Work out the finished part from the listing and answer in its coordinate system (mm). A direction names the side the tool comes from. Give positions to 0.01 mm unless a question says otherwise; leave off trailing zeros. Loops run counter-clockwise (first coordinate to the right, second up) from the corner with the lowest first, then second, coordinate; pieces in that order, holes last.
```python
from build123d import *

# Parameters (mm, degrees)
F0_W      = 60
F0_H      = 10
F1_DEPTH  = 60
F2_SIZE   = 9.99999
F9_DEPTH  = 40
F11_DEPTH = 20
F13_R     = 15
F14_DEPTH = 26
F15_R     = 2


# Not quite as in the source:
# - a fillet or chamfer is up to 0.001 mm smaller than in the source, because OpenCascade refuses the exact size


with BuildPart() as f1:
    # F0 (on Front) → F1 (new body)
    with BuildSketch(Plane.XZ):
        with Locations((30, 5)):
            Rectangle(F0_W, F0_H)
    extrude(amount=-F1_DEPTH)

    # F2 (size 10 in the source; OpenCascade refuses exactly that, so slightly less here)
    f2_edges = [f1.edges().sort_by_distance(p)[0] for p in [
        (60, 30, 0),
    ]]
    chamfer(f2_edges, length=F2_SIZE)

    # F5 (on face) → F6 section 0
    with BuildSketch(Plane.XY.offset(10), mode=Mode.PRIVATE) as f6_s0:
        Polygon((60, 0), (60, 60), (0, 0), align=None)
    loft([f6_s0.sketch, Vertex(60, 60, 70)])

    # F8 (on face) → F9 (join)
    with BuildSketch(Plane.XY.offset(10)):
        Polygon((40, 60), (0, 60), (0, 20), align=None)
    extrude(amount=F9_DEPTH)

    # F10 (on face) → F11 (join)
    with BuildSketch(Plane(origin=(0, 0, 0), x_dir=(1, 0, 0), z_dir=(0, 0, -1))):
        Polygon((0, -20), (0, -60), (40, -60), align=None)
    extrude(amount=F11_DEPTH)

    # F9_face (on face) → F12 section 0
    with BuildSketch(Plane(origin=(13.3333333333, 46.6666666667, 50), x_dir=(1, 0, 0), z_dir=(0, 0, 1)), mode=Mode.PRIVATE) as f12_s0:
        Polygon((26.6666666667, 13.3333333333), (-13.3333333333, 13.3333333333), (-13.3333333333, -26.6666666667), align=None)
    loft([f12_s0.sketch, Vertex(0, 60, -20)], mode=Mode.SUBTRACT)

    # F13 (on face) → F14 (cut)
    with BuildSketch(Plane(origin=(0, 0, -20), x_dir=(1, 0, 0), z_dir=(0, 0, -1))):
        with Locations((30, -40)):
            Circle(F13_R)
    extrude(amount=-F14_DEPTH, mode=Mode.SUBTRACT)

    # F15
    f15_edges = [f1.edges().sort_by_distance(p)[0] for p in [
        (15, 40, 6),
    ]]
    fillet(f15_edges, radius=F15_R)


solid = f1.part
```
Q1. Section C-C on x = 30 is taken. Give the vertices of the cut face in (y, z).
Q2. Consider line 1 along Y through (x, z) = (30, -13); line 2 along X through (y, z) = (22, 24.5); line 3 along Z through (x, y) = (12, 52). Determine where each line is inside the solid, lowest interval first.
Q3. Section A-A on y = 4 is taken. Give the vertices of the cut face in (x, z), plus the area to 3 significant figures.
Q4. Section D-D on z = 36.5 is taken. Give the vertices of the cut face in (x, y), plus the area to 3 significant figures.
Q5. Given pin 1 (4 mm diameter, centred on x = 30.5, y = 37.5, fed in from -Z); pin 2 (4 mm diameter, centred on x = 24, z = 14, fed in from -Y); pin 3 (12 mm diameter, centred on x = 19, z = 55, fed in from +Y), each flat-ended and moving along its own axis, determine where each tip first touches the part or whether it passes through.
Q6. Section B-B on z = 8 is taken. Give the vertices of the cut face in (x, y), plus the area to 3 significant figures.
Q7. Which of the six approach directions +Z, -Z, +X, -X, +Y, -Y give full straight-line access (tool end or side, diameter ignored) to faces 5 (the face through (8, 28, -10)), 6 (the face through (60, 43, 27)), 7 (the face through (43, 17, 27)), 8 (the face through (44, 44, 27)), 9 (the face through (18, 49, -6))?
Q8. Determine the mould class of faces 1 (the face through (0, 30, 8)), 2 (the face through (30, 0, 5)), 3 (the face through (30, 40, 6)), 4 (the face through (30, 60, 8)) for opening direction Y: +Y half, -Y half, draft (parallel to the pull), parting line (faces both ways), or undercut.
Check result:
1. outline: (0, 0) - (25, 0) - (25, 4) arc R2 cw to (27, 6) - (53, 6) arc R2 cw to (55, 4) - (55, -20) - (60, -20) - (60, 32.5) - (50, 50) - (50, 10) - (30, 10) - (30, 40) - (0, 10) - close
2. line 1: y = 55 to 60
2. line 2: x = 0 to 2, 22 to 60
2. line 3: z = -20 to 15
3. outline: (0, 0) - (50, 0) - (60, 10) - (60, 14) - (4, 14) - (4, 10) - (0, 10) - close
3. area: 774 mm2
4. outline: (0, 20) - (40, 60) - (32.29, 60) - (0, 27.71) - close; (26.5, 26.5) - (60, 26.5) - (60, 60) - close
4. area: 840 mm2
5. pin 1: stops at z = 6
5. pin 2: stops at y = 2
5. pin 3: stops at y = 42.32
6. outline: (0, 0) - (58, 0) - (58, 60) - (16, 60) - (0, 44) - close
6. area: 3,350 mm2
7. face 5: -Z, +X, -Y
7. face 6: +Z, -Z, +X, +Y, -Y
7. face 7: +Z, +X, -Y
7. face 8: +Z
7. face 9: -Z
8. face 1: draft
8. face 2: -Y half
8. face 3: undercut
8. face 4: +Y half
